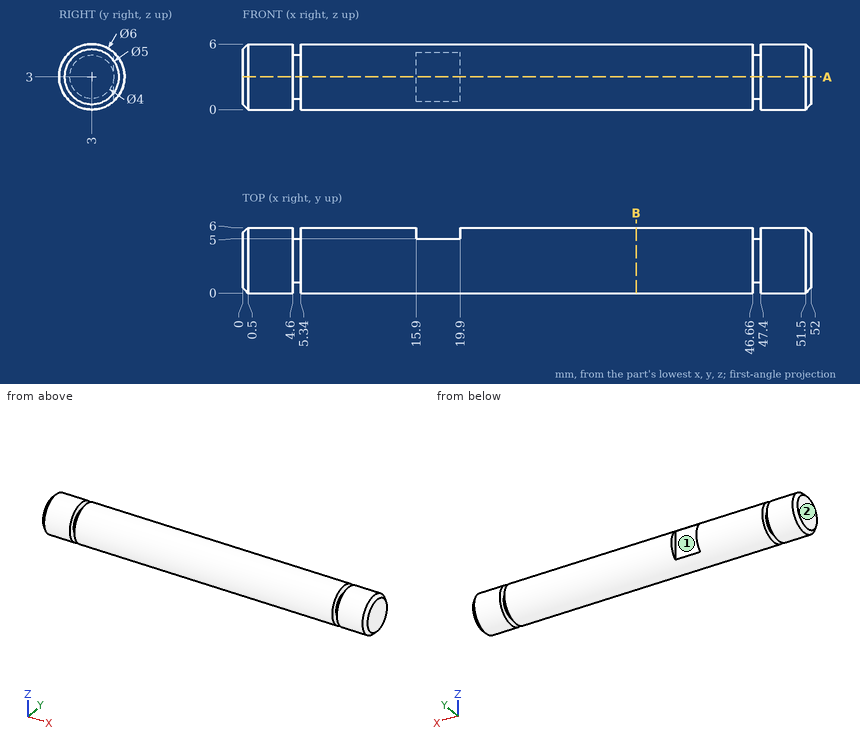
Print and shaded views of the part. All mm, measured from the part's lowest x, y and z. A direction names the side the tool comes from. Round coordinates to 2 decimals unless told otherwise and drop trailing zeros. Order: outer loops, then holes, each group sorted by start corner. A loop starts at its lowest first (then second) coordinate and runs counter-clockwise, first axis right, second up.
Q1. Drop flat-ended pins along their axis: pin 1 (1.2 mm diameter, centred on x = 18.5, z = 4, fed in from +Y); pin 2 (1.8 mm diameter, centred on y = 2.5, z = 4, fed in from -X); pin 3 (1.5 mm diameter, centred on x = 31, z = 4.5, fed in from -Y). Give the stop position or say it passes through.
Q2. Slice it at B-B (x = 36). Write the cut outline in (y, z), and give its area (3 significant figures).
Q3. Slice it at A-A (z = 3). Write the cut outline in (x, y), and give its area (3 significant figures).
Q4. Wall check: L1, parallel to X at y = 5.25, z = 1.75; L2, parallel to X at y = 4.75, z = 0.75; L3, parallel to X at y = 1.75, z = 0.5. Give the ranges that are in metal, low to high.
Q5. Which spindle directions (+Z, -Z, +X, -X, +Y, -Y) get a long thin tool onto all of the face, cutting with end or side? Do the marked faces 1 and 2. Say none if no direction does.
Results below:
1. pin 1: stops at y = 5
1. pin 2: stops at x = 0
1. pin 3: stops at y = 0.1
2. outline: circle Ø6 at (3, 3)
2. area: 28.3 mm2
3. outline: (0, 0.5) - (0.5, 0) - (4.6, 0) - (4.6, 1) - (5.34, 1) - (5.34, 0) - (46.66, 0) - (46.66, 1) - (47.4, 1) - (47.4, 0) - (51.5, 0) - (52, 0.5) - (52, 5.5) - (51.5, 6) - (47.4, 6) - (47.4, 5) - (46.66, 5) - (46.66, 6) - (19.9, 6) - (19.9, 5) - (15.9, 5) - (15.9, 6) - (5.34, 6) - (5.34, 5) - (4.6, 5) - (4.6, 6) - (0.5, 6) - (0, 5.5) - close
3. area: 305 mm2
4. L1: x = 0.07 to 4.6, 5.34 to 15.9, 19.9 to 46.66, 47.4 to 51.93
4. L2: x = 0.35 to 4.6, 5.34 to 46.66, 47.4 to 51.65
4. L3: x = 0.3 to 4.6, 5.34 to 46.66, 47.4 to 51.7
5. face 1: +Z, -Z, +Y
5. face 2: +Z, -Z, -X, +Y, -Y
